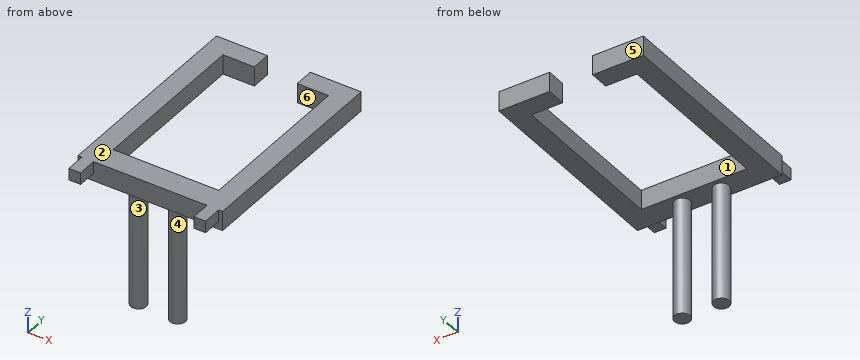
from build123d import *

# Parameters (mm, degrees)
SKETCH_1_W        = 3
SKETCH_1_H        = 3
EXTRUDE_1_DEPTH   = 5
EXTRUDE_1_2_DEPTH = 5
SKETCH_2_W        = 5
SKETCH_2_H        = 5
EXTRUDE_2_DEPTH   = 6
SKETCH_4_W        = 37
SKETCH_4_H        = 5
EXTRUDE_3_DEPTH   = 6
SKETCH_5_R        = 2
EXTRUDE_4_DEPTH   = 30
SKETCH_6_W        = 5
SKETCH_6_H        = 5
EXTRUDE_5_DEPTH   = 47
SKETCH_7_W        = 5
SKETCH_7_H        = 5
EXTRUDE_6_DEPTH   = 8
SKETCH_8_W        = 5
SKETCH_8_H        = 5
EXTRUDE_7_DEPTH   = 8


with BuildPart() as part:
    # Sketch 1 → Extrude 1 (new body)
    with BuildSketch(Plane(origin=(0, 0, 0), x_dir=(1, 0, 0), z_dir=(0, 1, 0))):
        with Locations((-301.650432081, -30.158642095)):
            Rectangle(SKETCH_1_W, SKETCH_1_H)
    extrude(amount=EXTRUDE_1_DEPTH)



with BuildPart() as body_2:
    # Sketch 1 → Extrude 1 2 (new body)
    with BuildSketch(Plane(origin=(0, 0, 0), x_dir=(1, 0, 0), z_dir=(0, 1, 0))):
        with Locations((-269.650432081, -30.158642095)):
            Rectangle(SKETCH_1_W, SKETCH_1_H)
    extrude(amount=EXTRUDE_1_2_DEPTH)


with BuildPart() as part_1:
    add(part.part)

    add(body_2.part)  # Extrude 2 merges body 2
    # Sketch 2 → Extrude 2 (add)
    with BuildSketch(Plane(origin=(0, 5, 0), x_dir=(1, 0, 0), z_dir=(0, 1, 0))):
        with Locations((-301.650432081, -29.158642095)):
            Rectangle(SKETCH_2_W, SKETCH_2_H)
        with Locations((-269.650432081, -29.158642095)):
            Rectangle(SKETCH_2_W, SKETCH_2_H)
    extrude(amount=EXTRUDE_2_DEPTH)

    # Sketch 4 → Extrude 3 (add)
    with BuildSketch(Plane(origin=(0, 11, 0), x_dir=(1, 0, 0), z_dir=(0, 1, 0))):
        with Locations((-285.650432081, -29.158642095)):
            Rectangle(SKETCH_4_W, SKETCH_4_H)
    extrude(amount=-EXTRUDE_3_DEPTH)

    # Sketch 5 → Extrude 4 (add)
    with BuildSketch(Plane(origin=(0, 0, 26.658642095), x_dir=(-1, 0, 0), z_dir=(0, 0, -1))):
        with Locations(Location((280.65047083, 8.019684887, 0), (0, 0, 180))):
            Circle(SKETCH_5_R)
        with Locations(Location((290.650393331, 7.980315113, 0), (0, 0, 180))):
            Circle(SKETCH_5_R)
    extrude(amount=EXTRUDE_4_DEPTH)

    # Sketch 6 → Extrude 5 (add)
    with BuildSketch(Plane(origin=(0, 11, 0), x_dir=(1, 0, 0), z_dir=(0, 1, 0))):
        with Locations((-269.650432081, -29.158642095)):
            Rectangle(SKETCH_6_W, SKETCH_6_H)
        with Locations((-301.650432081, -29.158642095)):
            Rectangle(SKETCH_6_W, SKETCH_6_H)
    extrude(amount=EXTRUDE_5_DEPTH)

    # Sketch 7 → Extrude 6 (add)
    with BuildSketch(Plane(origin=(-299.150432081, 0, 0), x_dir=(0, 0, -1), z_dir=(1, 0, 0))):
        with Locations((-29.158642095, 55.5)):
            Rectangle(SKETCH_7_W, SKETCH_7_H)
    extrude(amount=EXTRUDE_6_DEPTH)

    # Sketch 8 → Extrude 7 (add)
    with BuildSketch(Plane.ZY.offset(272.150432081)):
        with Locations((29.158642095, 55.5)):
            Rectangle(SKETCH_8_W, SKETCH_8_H)
    extrude(amount=EXTRUDE_7_DEPTH)


solid = part_1.part
Design review of the part built by this model. Coordinates are the model's own, in mm. Face numbers are marked on the shaded views. A direction names the side the tool comes from. Coordinates: 2 decimals unless noted, no trailing zeros. Order: outer loops, then holes, each group sorted by start corner. A loop starts at its lowest first (then second) coordinate and runs counter-clockwise, first axis right, second up. Notation, with made-up numbers: (48, 22) -> (72, 22) arc R18 ccw to (72, 36) -> close; hole circle Ø2 at (12.25, 59.25). An arc over 180 degrees is marked (long way). One line per item, written item: value.
1) We need section D-D, the plane z = 21.5. Give the boundary of the cut face in (x, y).
Output values:
outline: circle Ø4 at (-290.65, 7.98); circle Ø4 at (-280.65, 8.02)
2) Draft analysis for pull direction Y (two halves, no side actions). For the marked faces 1, 2 and 3, state which applies: +Y half, -Y half, draft (parallel to the pull), parting line (faces both ways), or undercut.
Output values:
face 1: undercut
face 2: draft
face 3: parting line
3) To check wall thickness, follow probe 1 along Z at (x, y) = (-299.5, 37.5); probe 2 along Y at (x, z) = (-289, 19.5); probe 3 along X at (y, z) = (9, 10.5). State the ranges of each line that lie inside material, in increasing order. Write a range as [from, to].
Output values:
probe 1: z = [26.66, 31.66]
probe 2: y = [6.85, 9.11]
probe 3: x = [-292.37, -288.93], [-282.39, -278.91]
4) Clearance check with flat-ended pins moving along their axes: P1, Ø1.5, axis at x = -269, y = 2.5, coming from the -Z side; P2, Ø1.5, axis at x = -284, z = 28.5, coming from the +Y side; P3, Ø5.5, axis at x = -296, z = 28.5, coming from the -Y side. State where each tip first meets the part, or that it passes through.
Output values:
P1: stops at z = 28.66
P2: stops at y = 11
P3: stops at y = 5
5) We need section A-A, the plane y = 20. Give the boundary of the cut face in (x, z).
Output values:
outline: (-304.15, 26.66) -> (-299.15, 26.66) -> (-299.15, 31.66) -> (-304.15, 31.66) -> close; (-272.15, 26.66) -> (-267.15, 26.66) -> (-267.15, 31.66) -> (-272.15, 31.66) -> close
6) Machinability: for the marked faces 4, 5 and 6, which of the approach directions +Z, -Z, +X, -X, +Y, -Y give a long, thin tool a straight path to every point of the face, cutting with its end or side? Answer none if there is none.
Output values:
face 4: -Z
face 5: +Z, -Z, +X, -X, +Y
face 6: +Z, -Z
7) We need section C-C, the plane x = -301. Give the boundary of the cut face in (y, z), then the cut area to 3 significant figures.
Output values:
outline: (0, 28.66) -> (5, 28.66) -> (5, 26.66) -> (58, 26.66) -> (58, 31.66) -> (0, 31.66) -> close
area: 280 mm2
8) We need section B-B, the plane x = -296. Give the boundary of the cut face in (y, z), then the cut area to 3 significant figures.
Output values:
outline: (5, 26.66) -> (11, 26.66) -> (11, 31.66) -> (5, 31.66) -> close; (53, 26.66) -> (58, 26.66) -> (58, 31.66) -> (53, 31.66) -> close
area: 55.0 mm2
